Input: dimensioned drawing with shaded views. Units: mm. Origin: part minimum x, y, z. A direction names the side the tool comes from. Coordinates: 2 decimals unless noted, no trailing zeros. Loops run counter-clockwise (first coordinate to the right, second up) from the corner with the lowest first, then second, coordinate; pieces in that order, holes last.
Item 1: Section B-B on x = 19.5. Return loops of the section in (y, z), and give its area (3 significant figures).
Item 2: Reachability of the marked faces 4, 5 and 6 from +Z, -Z, +X, -X, +Y, -Y: full face, straight path, thin tool, end or side. Return the list, or none.
Item 3: Contact query for flat-ended pins moving along their axis: P1, Ø2, axis at x = 18.5, y = 7.5, coming from the +Z side; P2, Ø4, axis at y = 5, z = 26.5, coming from the +X side; P3, Ø2, axis at x = 19.5, y = 6.5, coming from the +Z side. Output: stop coordinate, or through.
Item 4: Section D-D on z = 5.5. Return loops of the section in (x, y).
Item 5: Section C-C on y = 7.5. Return loops of the section in (x, z), and give its area (3 significant figures).
Item 6: Ray query, line 1 along Z through (x, y) = (17, 5.4); line 2 along Z through (x, y) = (17, 6.5); line 3 along Y through (x, z) = (32, 11.5). Return the intervals inside material, ascending.
Item 7: Section A-A on z = 17. Return loops of the section in (x, y), and give its area (3 significant figures).
Item 8: Pull-direction query (Z, two-part tool) for the marked faces 1, 2 and 3; classes: released by +Z, released by -Z, zero draft, split by the parting line, or undercut.
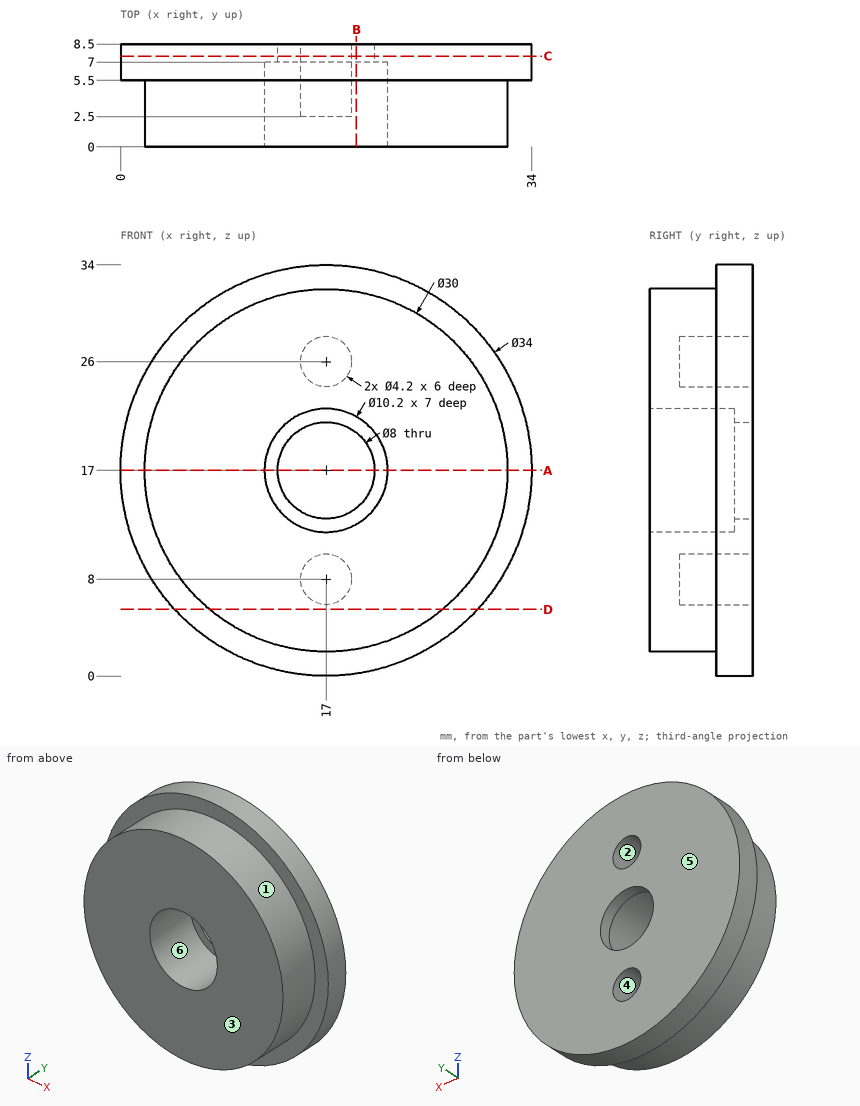
Results found:
1. outline: (0, 2.21) - (5.5, 2.21) - (5.5, 0.18) - (8.5, 0.18) - (8.5, 13.88) - (7, 13.88) - (7, 12.55) - (0, 12.55) - close; (0, 21.45) - (7, 21.45) - (7, 20.12) - (8.5, 20.12) - (8.5, 33.82) - (5.5, 33.82) - (5.5, 31.79) - (0, 31.79) - close
1. area: 192 mm2
2. face 4: +Y
2. face 5: +Z, -Z, +X, -X, +Y
2. face 6: -Y
3. P1: stops at z = 33.99
3. P2: stops at x = 32.22
3. P3: stops at z = 33.93
4. outline: (4.48, 5.5) - (7.37, 5.5) - (7.37, 0) - (26.63, 0) - (26.63, 5.5) - (29.52, 5.5) - (29.52, 8.5) - (4.48, 8.5) - close
5. outline: circle Ø34 at (17, 17); hole circle Ø8 at (17, 17); hole circle Ø4.2 at (17, 8); hole circle Ø4.2 at (17, 26)
5. area: 830 mm2
6. line 1: z = 2 to 5.9, 10.1 to 11.9, 22.1 to 23.9, 28.1 to 32
6. line 2: z = 0 to 5.9, 10.1 to 11.9, 22.1 to 23.9, 28.1 to 34
6. line 3: y = 5.5 to 8.5
7. outline: (0, 5.5) - (2, 5.5) - (2, 0) - (11.9, 0) - (11.9, 7) - (13, 7) - (13, 8.5) - (0, 8.5) - close; (21, 7) - (22.1, 7) - (22.1, 0) - (32, 0) - (32, 5.5) - (34, 5.5) - (34, 8.5) - (21, 8.5) - close
7. area: 184 mm2
8. face 1: split by the parting line
8. face 2: undercut
8. face 3: zero draft
